from build123d import *

# Parameters (mm, degrees)
F0_R     = 14.2875
F1_DEPTH = 25.4
F2_DEPTH = 15.89601


with BuildPart() as f1:
    # F0 (on Front) → F1 (new body)
    with BuildSketch(Plane.XZ):
        with BuildLine():
            Line((9.7499238233, 26.8601863441), (0, 28.575))
            ThreePointArc((0, 28.575), (-28.575, 0), (0, -28.575))
            Line((0, -28.575), (9.7818449028, -26.8485779008))
            ThreePointArc((9.7818449028, -26.8485779008), (23.4099000756, -16.3861894122), (28.575, 0))
            ThreePointArc((28.575, 0), (23.4001570321, 16.4000998739), (9.7499238233, 26.8601863441))
        make_face()
        with BuildLine():
            ThreePointArc((-13.4703841816, 4.7625), (0, 14.2875), (13.4703841816, 4.7625))
            Line((13.4703841816, 4.7625), (19.05, 4.7625))
            Line((19.05, 4.7625), (19.05, -4.7625))
            Line((19.05, -4.7625), (13.4703841816, -4.7625))
            ThreePointArc((13.4703841816, -4.7625), (0, -14.2875), (-13.4703841816, -4.7625))
            Line((-13.4703841816, -4.7625), (-19.05, -4.7625))
            Line((-19.05, -4.7625), (-19.05, 4.7625))
            Line((-19.05, 4.7625), (-13.4703841816, 4.7625))
        make_face(mode=Mode.SUBTRACT)
        with BuildLine():
            Line((54.1615282252, 19.0490867818), (9.7499238233, 26.8601863441))
            ThreePointArc((9.7499238233, 26.8601863441), (23.4001570321, 16.4000998739), (28.575, 0))
            ThreePointArc((28.575, 0), (23.4099000756, -16.3861894122), (9.7818449028, -26.8485779008))
            Line((9.7818449028, -26.8485779008), (53.9683106658, -19.0499988255))
            ThreePointArc((53.9683106658, -19.0499988255), (34.9252449744, 0.096609856), (54.1615282252, 19.0490867818))
        make_face()
        with BuildLine():
            ThreePointArc((73.025, 0), (67.5111712218, 13.4042742681), (54.1615282252, 19.0490867818))
            ThreePointArc((54.1615282252, 19.0490867818), (34.9252449744, 0.096609856), (53.9683106658, -19.0499988255))
            ThreePointArc((53.9683106658, -19.0499988255), (67.4430189372, -13.4727490108), (73.025, 0))
        make_face()
        with Locations((53.975, 0)):
            Circle(F0_R, mode=Mode.SUBTRACT)
        with BuildLine():
            ThreePointArc((-13.4703841816, -4.7625), (-14.2875, 0), (-13.4703841816, 4.7625))
            Line((-13.4703841816, 4.7625), (-19.05, 4.7625))
            Line((-19.05, 4.7625), (-19.05, -4.7625))
            Line((-19.05, -4.7625), (-13.4703841816, -4.7625))
        make_face()
    extrude(amount=F1_DEPTH)

    # F0 (on Front) → F2 (join)
    with BuildSketch(Plane.XZ):
        with BuildLine():
            Line((9.7499238233, 26.8601863441), (0, 28.575))
            ThreePointArc((0, 28.575), (-28.575, 0), (0, -28.575))
            Line((0, -28.575), (9.7818449028, -26.8485779008))
            ThreePointArc((9.7818449028, -26.8485779008), (23.4099000756, -16.3861894122), (28.575, 0))
            ThreePointArc((28.575, 0), (23.4001570321, 16.4000998739), (9.7499238233, 26.8601863441))
        make_face()
        with BuildLine():
            ThreePointArc((-13.4703841816, 4.7625), (0, 14.2875), (13.4703841816, 4.7625))
            Line((13.4703841816, 4.7625), (19.05, 4.7625))
            Line((19.05, 4.7625), (19.05, -4.7625))
            Line((19.05, -4.7625), (13.4703841816, -4.7625))
            ThreePointArc((13.4703841816, -4.7625), (0, -14.2875), (-13.4703841816, -4.7625))
            Line((-13.4703841816, -4.7625), (-19.05, -4.7625))
            Line((-19.05, -4.7625), (-19.05, 4.7625))
            Line((-19.05, 4.7625), (-13.4703841816, 4.7625))
        make_face(mode=Mode.SUBTRACT)
        with BuildLine():
            ThreePointArc((-13.4703841816, -4.7625), (-14.2875, 0), (-13.4703841816, 4.7625))
            Line((-13.4703841816, 4.7625), (-19.05, 4.7625))
            Line((-19.05, 4.7625), (-19.05, -4.7625))
            Line((-19.05, -4.7625), (-13.4703841816, -4.7625))
        make_face()
    extrude(amount=-F2_DEPTH)


solid = f1.part
Build history of the part. All positions in model axes, mm. A direction names the side the tool comes from. Give positions to 0.01 mm unless a question says otherwise; leave off trailing zeros. Order: outer loops, then holes, each group sorted by start corner. A loop starts at its lowest first (then second) coordinate and runs counter-clockwise, first axis right, second up. Notation, with made-up numbers: M 22,40.25 L 55,40.25 A28 ccw 55,69.25 Z; hole C 28,39 d11. An arc over 180 degrees is marked long. Put each result on its own line as item: value.
Item 1: Drop flat-ended pins along their axis: pin 1 Ø8 at (x, y) = (27.5, -11.5) entering from -Z; pin 2 Ø6 at (x, y) = (16, -13.5) entering from +Z; pin 3 Ø4.5 at (x, y) = (17.5, -14) entering from -Z. Give the stop position or say it passes through.
Results are:
pin 1: z = -24.43
pin 2: z = 26.29
pin 3: z = -25.88
Item 2: Which spindle directions (+Z, -Z, +X, -X, +Y, -Y) get a long thin tool onto all of the face, cutting with end or side? Do faces 4 (the face through (16, -5, 4.762)), 5 (the face through (-13, 15.896, 7)). Say none if no direction does.
Results are:
face 4: +Y, -Y
face 5: +Z, -Z, +X, -X, +Y
Item 3: Cut at C-C on x = 1.5. Write the cut outline in (y, z).
Results are:
outline: M -25.4,-28.31 L 15.9,-28.31 L 15.9,-14.21 L -25.4,-14.21 Z; M -25.4,14.21 L 15.9,14.21 L 15.9,28.31 L -25.4,28.31 Z
Item 4: Cut at D-D on x = 45.5. Write the cut outline in (y, z).
Results are:
outline: M -25.4,-20.54 L 0,-20.54 L 0,-11.5 L -25.4,-11.5 Z; M -25.4,11.5 L 0,11.5 L 0,20.57 L -25.4,20.57 Z
Item 5: Cut at B-B on z = 12.5. Write the cut outline in (x, y), then the cut area to 3 significant figures.
Results are:
outline: M -25.7,-25.4 L -6.92,-25.4 L -6.92,15.9 L -25.7,15.9 Z; M 6.92,-25.4 L 47.06,-25.4 L 47.06,0 L 25.7,0 L 25.7,15.9 L 6.92,15.9 Z; M 60.89,-25.4 L 68.35,-25.4 L 68.35,0 L 60.89,0 Z
area: 2,280 mm2
Item 6: Wall check: probe 1 along X at (y, z) = (-20, -4.5); probe 2 along Y at (x, z) = (33, -12.5); probe 3 along X at (y, z) = (2, -0.5). Give the ranges that are in metal, low to high.
Results are:
probe 1: -28.22 to -13.56, 19.05 to 40.41, 67.54 to 72.49
probe 2: -25.4 to 0
probe 3: -28.57 to -14.28, 19.05 to 28.57
Item 7: Pull direction Z, two halves, no side cores. Call faces 1 (the face through (-28.57, -5.04, 0.63)), 2 (the face through (39, 0, -2)), 3 (the face through (16, -5, -4.762)): +Z half, -Z half, draft (parallel to the pull), parting line (faces both ways), or undercut.
Results are:
face 1: parting line
face 2: draft
face 3: undercut
Item 8: Cut at A-A on y = -14.5. Count the separate pieces of the cut face and the enclosed holes in it, then the cut area to 3 significant figures.
Results are:
separate pieces: 1
enclosed holes: 2
area: 3,090 mm2
